For this review, take the finished solid that the model builds, in its own axes (mm). A direction names the side the tool comes from. Give positions to 0.01 mm unless a question says otherwise; leave off trailing zeros. Loops run counter-clockwise (first coordinate to the right, second up) from the corner with the lowest first, then second, coordinate; pieces in that order, holes last.
```python
from build123d import *

# Parameters (mm, degrees)
F0_R     = 18.3
F0_R_2   = 16.8
F1_DEPTH = 83.6
F3_R     = 18.3
F3_R_2   = 16.8
F4_DEPTH = 23
F5_DEPTH = 18.8
F6_R     = 18.3
F6_R_2   = 16.8
F7_DEPTH = 18.8
F8_R     = 16.5
F9_DEPTH = 102.5


with BuildPart() as f1:
    # F0 (on Top) → F1 (new body)
    with BuildSketch(Plane.XY):
        Circle(F0_R)
        Circle(F0_R_2, mode=Mode.SUBTRACT)
    extrude(amount=F1_DEPTH)

    # F3 (on offset) → F5 (cut)
    with BuildSketch(Plane.XZ.offset(18.8)):
        with Locations((0, 41.8)):
            Circle(F3_R)
        with Locations((0, 41.8)):
            Circle(F3_R_2, mode=Mode.SUBTRACT)
        with Locations((0, 41.8)):
            Circle(F3_R_2)
    extrude(amount=-F5_DEPTH, mode=Mode.SUBTRACT)



with BuildPart() as f4:
    # F3 (on offset) → F4 (new body)
    with BuildSketch(Plane.XZ.offset(18.8)):
        with Locations((0, 41.8)):
            Circle(F3_R)
        with Locations((0, 41.8)):
            Circle(F3_R_2, mode=Mode.SUBTRACT)
    extrude(amount=F4_DEPTH)


with BuildPart() as f1_1:
    add(f1.part)

    add(f4.part)  # F7 merges F4
    # F6 (on face) → F7 (join)
    with BuildSketch(Plane(origin=(0, -18.8, 0), x_dir=(-1, 0, 0), z_dir=(0, 1, 0))):
        with Locations((0, 41.8)):
            Circle(F6_R)
        with Locations((0, 41.8)):
            Circle(F6_R_2, mode=Mode.SUBTRACT)
    extrude(amount=F7_DEPTH)

    # F8 (on face) → F9 (cut)
    with BuildSketch(Plane(origin=(0, 0, 0), x_dir=(1, 0, 0), z_dir=(0, 0, -1))):
        Circle(F8_R)
    extrude(amount=-F9_DEPTH, mode=Mode.SUBTRACT)


solid = f1_1.part
```
Item 1: Take a section at C-C on z = 46. Give the boundary of the cut face in (x, y), and give its area (3 significant figures).
Answer:
outline: (-17.81, -41.8) - (-16.27, -41.8) - (-16.27, -2.77) arc R16.5 cw to (-16.5, 0) - (-16.8, 0) arc R16.8 cw to (16.8, 0) - (16.5, 0) arc R16.5 cw to (16.27, -2.77) - (16.27, -41.8) - (17.81, -41.8) - (17.81, -4.2) arc R18.3 ccw (long way) to (-17.81, -4.2) - close
area: 214 mm2
Item 2: Take a section at D-D on x = -8.5. Give the boundary of the cut face in (y, z).
Answer:
outline: (-41.8, 25.59) - (-16.21, 25.59) - (-16.21, 0) - (-14.49, 0) - (-14.49, 25.59) - (-14.14, 25.59) - (-14.14, 27.31) - (-41.8, 27.31) - close; (-41.8, 56.29) - (-14.14, 56.29) - (-14.14, 58.01) - (-14.49, 58.01) - (-14.49, 83.6) - (-16.21, 83.6) - (-16.21, 58.01) - (-41.8, 58.01) - close; (14.49, 0) - (16.21, 0) - (16.21, 83.6) - (14.49, 83.6) - close
Item 3: Take a section at B-B on y = -11.5. Give the boundary of the cut face in (x, z).
Answer:
outline: (-14.24, 0) - (-12.25, 0) - (-12.25, 28.2) arc R18.3 ccw to (-11.83, 27.84) - (-11.83, 29.87) arc R16.8 cw to (-11.83, 53.73) - (-11.83, 55.76) arc R18.3 ccw to (-12.25, 55.4) - (-12.25, 83.6) - (-14.24, 83.6) - (-14.24, 53.3) arc R18.3 ccw to (-14.24, 30.3) - close; (11.83, 27.84) arc R18.3 ccw to (12.25, 28.2) - (12.25, 0) - (14.24, 0) - (14.24, 30.3) arc R18.3 ccw to (14.24, 53.3) - (14.24, 83.6) - (12.25, 83.6) - (12.25, 55.4) arc R18.3 ccw to (11.83, 55.76) - (11.83, 53.73) arc R16.8 cw to (11.83, 29.87) - close
Item 4: Clearance check with flat-ended pins moving along their axes: pin 1 Ø8 at (y, z) = (-26, 60.5) entering from +X; pin 2 Ø20 at (x, z) = (0, 41.8) entering from -Y; pin 3 Ø12 at (y, z) = (5, 67) entering from -X; pin 4 Ø2 at (y, z) = (-21, 74) entering from +X. State where each tip first meets the part, or that it passes through.
Answer:
pin 1: stops at x = 10.9
pin 2: stops at y = 13.5
pin 3: stops at x = -18.3
pin 4: passes through
Item 5: Tool access review of faces 4 (the cylindrical face through (2.036, -16.374, 24.866)), 5 (the flat face through (16, -41.8, 36)), 6 (the cylindrical face through (-2.187, 16.657, 41.215)): name each direction out of +Z, -Z, +X, -X, +Y, -Y from which nothing blocks a thin tool from reaching the whole face with its end or side.
Answer:
face 4: +Z, -Z
face 5: +Z, -Z, +X, -X, -Y
face 6: none
Item 6: For L1, parallel to Y at x = 0, z = 17.5; L2, parallel to X at y = -14.5, z = 41; L3, parallel to Y at x = -12, z = 16.5, list the stretches that pass through material, from the lowest coordinate up.
Answer:
L1: y = -18.3 to -16.8, 16.8 to 18.3
L2: x = -18.28 to -16.78, 16.78 to 18.28
L3: y = -13.82 to -11.76, 11.76 to 13.82
Item 7: The part is to be moulded in two halves that separate along Y. For faces 1 (the cylindrical face through (-2.382, 18.144, 41.215)), 2 (the cylindrical face through (2.036, -16.374, 58.663)), 3 (the flat face through (8, -15, 83.6)), say which applies: released by +Y, released by -Y, zero draft, split by the parting line, or undercut.
Answer:
face 1: split by the parting line
face 2: undercut
face 3: zero draft
Item 8: Take a section at A-A on x = 0. Give the boundary of the cut face in (y, z).
Answer:
outline: (-41.8, 23.5) - (-18.3, 23.5) - (-18.3, 0) - (-16.8, 0) - (-16.8, 23.5) - (-16.5, 23.5) - (-16.5, 25) - (-41.8, 25) - close; (-41.8, 58.6) - (-16.5, 58.6) - (-16.5, 60.1) - (-16.8, 60.1) - (-16.8, 83.6) - (-18.3, 83.6) - (-18.3, 60.1) - (-41.8, 60.1) - close; (16.8, 0) - (18.3, 0) - (18.3, 83.6) - (16.8, 83.6) - close
